```python
from build123d import *
from build123d.topology import SkipClean

# Parameters (mm, degrees)
SKETCH1_W           = 40.5
SKETCH1_H           = 20
BOSS_EXTRUDE1_DEPTH = 26.9
BOSS_EXTRUDE2_DEPTH = 5
SKETCH3_R           = 1.5
CUT_EXTRUDE1_DEPTH  = 67.10491661


with BuildPart() as part:
    # Sketch1 → Boss-Extrude1 (new body)
    with BuildSketch(Plane(origin=(0, 0, 0), x_dir=(1, 0, 0), z_dir=(0, 1, 0))):
        Polygon((0, 0), (0, 28), (48.5, 28), (48.5, 0), (38.5, -10), (48.5, -20), (48.5, -23), (0, -23), (0, -20), (10, -10), align=None)
        with Locations((24.25, 14)):
            Rectangle(SKETCH1_W, SKETCH1_H, mode=Mode.SUBTRACT)
        Polygon((3, 0), (20, 0), (11.5, -8.5), align=None, mode=Mode.SUBTRACT)
        Polygon((13, -10), (23, 0), (25.5, 0), (35.5, -10), (25.5, -20), (23, -20), align=None, mode=Mode.SUBTRACT)
        Polygon((11.5, -11.5), (3, -20), (20, -20), align=None, mode=Mode.SUBTRACT)
        Polygon((45.5, 0), (28.5, 0), (37, -8.5), align=None, mode=Mode.SUBTRACT)
        Polygon((37, -11.5), (28.5, -20), (45.5, -20), align=None, mode=Mode.SUBTRACT)
    extrude(amount=BOSS_EXTRUDE1_DEPTH)

    # Sketch2 → Boss-Extrude2 (add)
    with BuildSketch(Plane(origin=(0, 26.9, 0), x_dir=(1, 0, 0), z_dir=(0, 1, 0))):
        with BuildLine():
            Line((-5, 0), (0, 0))
            Line((0, 0), (0, 7.55))
            ThreePointArc((0, 7.55), (-1.5, 9.05), (0, 10.55))
            Line((0, 10.55), (0, 17.45))
            ThreePointArc((0, 17.45), (-1.5, 18.95), (0, 20.45))
            Line((0, 20.45), (0, 28))
            Line((0, 28), (-5, 28))
            Line((-5, 28), (-5, 0))
        make_face()
        with BuildLine():
            Line((53.5, 28), (48.5, 28))
            Line((48.5, 28), (48.5, 20.45))
            ThreePointArc((48.5, 20.45), (50, 18.95), (48.5, 17.45))
            Line((48.5, 17.45), (48.5, 10.55))
            ThreePointArc((48.5, 10.55), (50, 9.05), (48.5, 7.55))
            Line((48.5, 7.55), (48.5, 0))
            Line((48.5, 0), (53.5, 0))
            Line((53.5, 0), (53.5, 28))
        make_face()
    extrude(amount=-BOSS_EXTRUDE2_DEPTH)

    # Sketch3 → Cut-Extrude1 (cut, through all)
    with SkipClean():  # the faces are left unmerged after this step: merging them gives an invalid solid
        with BuildSketch(Plane(origin=(0, 26.9, 0), x_dir=(1, 0, 0), z_dir=(0, 1, 0))):
            with Locations(Location((0, 18.95, 0), (0, 0, 270))):
                Circle(SKETCH3_R)
            with Locations(Location((0, 9.05, 0), (0, 0, 270))):
                Circle(SKETCH3_R)
            with Locations(Location((48.5, 9.05, 0), (0, 0, 270))):
                Circle(SKETCH3_R)
            with Locations(Location((48.5, 18.95, 0), (0, 0, 270))):
                Circle(SKETCH3_R)
        extrude(amount=-CUT_EXTRUDE1_DEPTH, mode=Mode.SUBTRACT)


solid = part.part
```
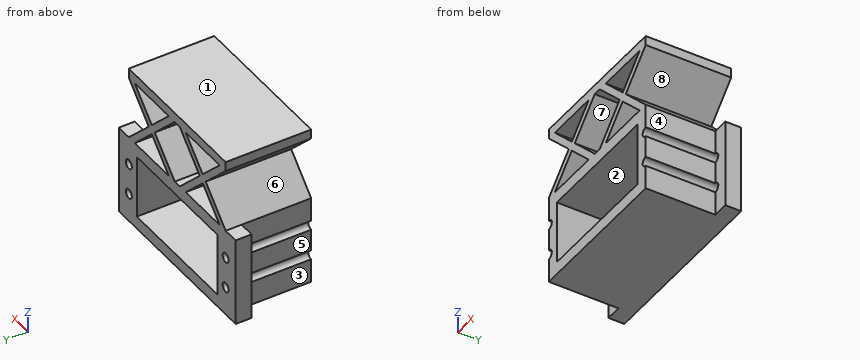
The listing builds one solid part. Answer for the finished solid, in the listing's coordinates (mm). Face numbers are marked on the shaded views. A direction names the side the tool comes from. Round coordinates to 2 decimals unless told otherwise and drop trailing zeros. Loops run counter-clockwise (first coordinate to the right, second up) from the corner with the lowest first, then second, coordinate; pieces in that order, holes last. Notation, with made-up numbers: (7.5, -19) - (51.5, -19) arc R24 ccw to (51.5, -8) - close; hole circle Ø7 at (8, -11). An arc over 180 degrees is marked (long way). Use one line per item in the form item = value. Start each with the question number.
1. Consider line 1 (Z direction, x = 25.5, y = 13); line 2 (X direction, y = 2.75, z = -6.5); line 3 (X direction, y = 13, z = -9.05). Determine where each line is inside the solid, lowest interval first. Write a range as [from, to].
2. The part is cut by section A-A on x = 43. Determine the outline of the cut face in (y, z).
3. The part is cut by section D-D on y = 25.25. Give the number of separate pieces and of enclosed holes in the cut face, then the cut area to 3 significant figures.
4. A tool of negligible diameter and unlimited length cuts with its end or side. For the marked faces 4, 5, 6, 7 and 8, from which of +Z, -Z, +X, -X, +Y, -Y can it reach the whole face along a straight path? Write none if from no direction.
5. The part is cut by section C-C on z = -5. Determine the outline of the cut face in (x, y).
6. The part is cut by section B-B on z = -18.95. Determine the outline of the cut face in (x, y), then the cut area to 4 significant figures.
7. Given pin 1 Ø6 at (y, z) = (13.5, -9.5) entering from +X; pin 2 Ø3 at (y, z) = (16, 10.5) entering from +X; pin 3 Ø1.5 at (x, y) = (-3.5, 23) entering from +Z, each flat-ended and moving along its own axis, determine where each tip first touches the part or whether it passes through.
8. For a pull along X with two mould halves and no side action, classify the marked faces 1, 2 and 3 as pulls with the +X half, pulls with the -X half, needs draft (parallel to the pull), parting line crosses it, or undercut.
Geometry check:
q1.line_1 = [-28, -24], [-4, 0], [20, 23]
q1.line_2 = [0, 4], [44.5, 48.5]
q1.line_3 = [1.5, 4], [44.5, 47]
q2.outline = (0, -28) - (26.9, -28) - (26.9, -24) - (0, -24) - close; (0, -4) - (26.9, -4) - (26.9, 0) - (0, 0) - close; (0, 2.5) - (26.9, 2.5) - (26.9, 5.5) - (0, 5.5) - close; (0, 14.5) - (26.9, 14.5) - (26.9, 17.5) - (0, 17.5) - close; (0, 20) - (26.9, 20) - (26.9, 23) - (0, 23) - close
q3.separate_pieces = 1
q3.enclosed_holes = 10
q3.area = 1,180 mm^2
q4.face_4 = +Z, -Z, +X, -Y
q4.face_5 = +Z, -Z, -X, -Y
q4.face_6 = -X, +Y, -Y
q4.face_7 = +Y, -Y
q4.face_8 = +X, +Y, -Y
q5.outline = (-5, 21.9) - (0, 21.9) - (0, 0) - (4, 0) - (4, 26.9) - (-5, 26.9) - close; (44.5, 0) - (48.5, 0) - (48.5, 21.9) - (53.5, 21.9) - (53.5, 26.9) - (44.5, 26.9) - close
q6.outline = (-5, 21.9) - (-1.5, 21.9) - (-1.5, 26.9) - (-5, 26.9) - close; (1.5, 0) - (4, 0) - (4, 26.9) - (1.5, 26.9) - close; (44.5, 0) - (47, 0) - (47, 26.9) - (44.5, 26.9) - close; (50, 21.9) - (53.5, 21.9) - (53.5, 26.9) - (50, 26.9) - close
q6.area = 169.5 mm^2
q7.pin_1 = 48.5
q7.pin_2 = 40.5
q7.pin_3 = 0
q8.face_1 = needs draft
q8.face_2 = undercut
q8.face_3 = pulls with the -X half
